```python
from build123d import *

# Parameters (mm, degrees)
CROQUIS1_W              = 34
CROQUIS1_H              = 22
CROQUIS1_R              = 7.5
SALIENTE_EXTRUIR1_DEPTH = 30
CROQUIS2_R              = 2
CORTAR_EXTRUIR1_DEPTH   = 30
CHAFL_N1_SIZE           = 3


with BuildPart() as part:
    # Croquis1 → Saliente-Extruir1 (new body)
    with BuildSketch(Plane.XY):
        with Locations((0, -11)):
            Rectangle(CROQUIS1_W, CROQUIS1_H)
        with Locations((0, -11)):
            Circle(CROQUIS1_R, mode=Mode.SUBTRACT)
    extrude(amount=SALIENTE_EXTRUIR1_DEPTH)

    # Croquis2 → Cortar-Extruir1 (cut)
    with BuildSketch(Plane(origin=(0, 0, 0), x_dir=(1, 0, 0), z_dir=(0, 1, 0))):
        with Locations(Location((-12, -6, 0), (0, 0, 270))):
            Circle(CROQUIS2_R)
        with Locations(Location((12, -6, 0), (0, 0, 270))):
            Circle(CROQUIS2_R)
        with Locations(Location((-12, -24, 0), (0, 0, 270))):
            Circle(CROQUIS2_R)
        with Locations(Location((12, -24, 0), (0, 0, 270))):
            Circle(CROQUIS2_R)
    extrude(amount=-CORTAR_EXTRUIR1_DEPTH, mode=Mode.SUBTRACT)

    # Chaflán1
    chafl_n1_edges = [part.edges().sort_by_distance(p)[0] for p in [
        (17, -22, 15),
        (-17, -22, 15),
        (-17, 0, 15),
        (17, 0, 15),
    ]]
    chamfer(chafl_n1_edges, length=CHAFL_N1_SIZE - 0.0001)  # a hair under: the kernel refuses the full size


solid = part.part
```
Design review of the part built by this model. Coordinates are the model's own, in mm. Coordinates: 2 decimals unless noted, no trailing zeros. Write each loop counter-clockwise with the first axis right and the second up, starting at its lowest first coordinate (ties: lowest second). Pieces come first, ordered by that corner, then holes.
1) Mouldability with a two-part tool opening along Z and no side actions: class faces 1 (the cylindrical face through (14, -11, 24)), 2 (the flat face through (-15, -21, 15)), 3 (the flat face through (-8, -11, 30)) as +Z half, -Z half, draft (parallel to the pull), parting line (faces both ways), or undercut.
2) Add section A-A (z = 24). State how many separate pieces and enclosed holes the cut face has, plus the area to 3 significant figures.
3) To check wall thickness, follow L1, parallel to X at y = -11.25, z = 6; L2, parallel to X at y = -7.5, z = 24; L3, parallel to Y at x = 0, z = 12. State the ranges of each line that lie inside material, in increasing order.
4) Add section B-B (y = -11). Write out the cut boundary in (x, z).
5) Add section C-C (x = 0). Write out the cut boundary in (y, z).
6) Add section D-D (z = 2.5). Write out the cut boundary in (x, y), plus the area to 3 significant figures.
7) Insertion check: pin 1 (5 mm diameter, centred on x = -12, z = 24, fed in from -Y). The pin has a flat end and moves straight along its axis. Give the tip position at first contact, or say it passes through.
Check result:
1. face 1: undercut
1. face 2: draft
1. face 3: +Z half
2. separate pieces: 3
2. enclosed holes: 1
2. area: 377 mm2
3. L1: x = -17 to -14, -10 to -7.5, 7.5 to 10, 14 to 17
3. L2: x = -17 to -14, -10 to -6.63, 6.63 to 10, 14 to 17
3. L3: y = -22 to -18.5, -3.5 to 0
4. outline: (-17, 0) - (-7.5, 0) - (-7.5, 30) - (-17, 30) - close; (7.5, 0) - (17, 0) - (17, 30) - (7.5, 30) - close; hole circle Ø4 at (-12, 6); hole circle Ø4 at (-12, 24); hole circle Ø4 at (12, 6); hole circle Ø4 at (12, 24)
5. outline: (-22, 0) - (-18.5, 0) - (-18.5, 30) - (-22, 30) - close; (-3.5, 0) - (0, 0) - (0, 30) - (-3.5, 30) - close
6. outline: (-17, -19) - (-14, -22) - (14, -22) - (17, -19) - (17, -3) - (14, 0) - (-14, 0) - (-17, -3) - close; hole circle Ø15 at (0, -11)
6. area: 553 mm2
7. pin 1: stops at y = -22
